The listing builds one solid part. Answer for the finished solid, in the listing's coordinates (mm). A direction names the side the tool comes from. Give positions to 0.01 mm unless a question says otherwise; leave off trailing zeros. Order: outer loops, then holes, each group sorted by start corner. A loop starts at its lowest first (then second) coordinate and runs counter-clockwise, first axis right, second up. Notation, with made-up numbers: (26, 9) - (78, 9) arc R27 ccw to (78, 40) - close; hole circle Ø8 at (-9, 77.25). An arc over 180 degrees is marked (long way). Write each question's results on one line, items separated by ' | '. Start each with the question number.
1. Section C-C (z = 4.5) is taken. State how many separate pieces and enclosed holes the cut face has, and give its area (3 significant figures).
2. Section A-A (y = -37.5) is taken. Give the vertices of the cut face in (x, z), and give its area (3 significant figures).
3. A flat-ended cylindrical pin translates along its axis: pin 1 (4 mm diameter, centred on x = 38.5, y = 34.5, fed in from +Z). Find the tip coordinate at first contact, or state that the pin passes through.
4. Determine the mould class of faces 1 (the face through (-67.5, -1, 4)), 2 (the face through (37, 33, 3)), 3 (the face through (64.65, 64.49, 4.06)), 4 (the face through (37, -42, 3)) for opening direction X: released by +X, released by -X, zero draft, split by the parting line, or undercut.
5. Which of the six approach directions +Z, -Z, +X, -X, +Y, -Y give full straight-line access (tool end or side, diameter ignored) to faces 5 (the face through (-43.994, -37.214, 5.535)), 6 (the face through (1, -67.5, 4))?
6. Find the intervals of material crossed by L1, parallel to X at y = -37.5, z = 1.1; L2, parallel to Y at x = -37.5, z = 6.6, in increasing order.
Autodesk Inventor part; units mm, degrees
ref_plane "YZ Plane" through (0, 0, 0) normal (1, 0, 0) x (0, 1, 0)
ref_plane "XZ Plane" through (0, 0, 0) normal (0, 1, 0) x (-1, 0, 0)
ref_plane "XY Plane" through (0, 0, 0) normal (0, 0, 1) x (1, 0, 0)
sketch "Sketch1" plane through (0, 0, 0) normal (0, 0, 1) x (1, 0, 0)
  circle A0 centre (-57, 57.5) radius 3
  circle A1 centre (57, 57.5) radius 3
  circle A2 centre (-57, -57.5) radius 3
  circle A3 centre (57, -57.5) radius 3
  line L0 (-57, 57.5) -> (57, -57.5) construction
  line L1 (-57, -57.5) -> (57, 57.5) construction
  line L2 (-67.5, 67.5) -> (67.5, 67.5)
  line L3 (67.5, 67.5) -> (67.5, -67.5)
  line L4 (67.5, -67.5) -> (-67.5, -67.5)
  line L5 (-67.5, -67.5) -> (-67.5, 67.5)
  line L6 (-67.5, 67.5) -> (67.5, -67.5) construction
  line L7 (67.5, 67.5) -> (-67.5, -67.5) construction
  circle A4 centre (-37.5, 37.5) radius 4
  circle A5 centre (-37.5, -37.5) radius 4
  circle A6 centre (37.5, -37.5) radius 4
  circle A7 centre (37.5, 37.5) radius 4
  point P0 (0, 0)
  point P1 (0, 0)
  dimension "d0" = 114
  dimension "d1" = 115
  dimension "d2" = 6
  dimension "d3" = 135
  dimension "d4" = 135
  dimension "d5" = 8
  dimension "d6" = 30
  dimension "d9" = 360
extrude "Extrusion1" add sketch "Sketch1" along normal blind 8
sketch "Sketch2" plane through (0, 0, 8) normal (0, 0, 1) x (1, 0, 0)
  line L0 (-67.5, -67.5) -> (67.5, -67.5)
  line L1 (67.5, -67.5) -> (67.5, 67.5)
  line L2 (67.5, 67.5) -> (-67.5, 67.5)
  line L3 (-67.5, 67.5) -> (-67.5, -67.5)
  circle A0 centre (37.5, 37.5) radius 4
  circle A1 centre (37.5, -37.5) radius 4
  circle A2 centre (-37.5, -37.5) radius 4
  circle A3 centre (-37.5, 37.5) radius 4
  circle A4 centre (57, -57.5) radius 3
  circle A5 centre (-57, -57.5) radius 3
  circle A6 centre (57, 57.5) radius 3
  circle A7 centre (-57, 57.5) radius 3
  circle A8 centre (-37.5, 37.5) radius 6.5
  circle A9 centre (-37.5, -37.5) radius 6.5
  circle A10 centre (37.5, -37.5) radius 6.5
  circle A11 centre (37.5, 37.5) radius 6.5
  point P0 (0, 0)
  dimension "d13" = 13
  dimension "d16" = 360
extrude "Extrusion2" cut sketch "Sketch2" against normal blind 5 contours A0 | A1 | A2 | A3 | A8 | A9 | A10 | A11
fillet "Fillet1" radius 10 4 edges at (-67.5, 67.5, 4) (67.5, 67.5, 4) (-67.5, -67.5, 4) (67.5, -67.5, 4)
thread "Thread1"
thread "Thread2"
thread "Thread3"
thread "Thread4"
properties part number "plaat aan stoel" material "Aluminum 6061"
Reported:
1) separate pieces: 1 | enclosed holes: 8 | area: 17,500 mm²
2) outline: (-67.5, 0) - (-41.5, 0) - (-41.5, 3) - (-44, 3) - (-44, 8) - (-67.5, 8) - close; (-33.5, 0) - (33.5, 0) - (33.5, 3) - (31, 3) - (31, 8) - (-31, 8) - (-31, 3) - (-33.5, 3) - close; (41.5, 0) - (67.5, 0) - (67.5, 8) - (44, 8) - (44, 3) - (41.5, 3) - close | area: 902 mm²
3) pin 1: z = 3
4) face 1: released by -X | face 2: undercut | face 3: released by +X | face 4: undercut
5) face 5: +Z | face 6: +Z, -Z, +X, -X, -Y
6) L1: -67.5 to -41.5, -33.5 to 33.5, 41.5 to 67.5 | L2: -67.5 to -44, -31 to 31, 44 to 67.5
